```python
from build123d import *

# Parameters (mm, degrees)
SKETCH2_R            = 25
BOSS_EXTRUDE1_DEPTH  = 10
SKETCH3_R            = 20
BOSS_EXTRUDE2_DEPTH  = 8
BOSS_EXTRUDE3_DEPTH  = 20
SKETCH5_R            = 12.5
CUT_EXTRUDE1_DEPTH   = 52.903757089
CUT_SWEEP1_PROFILE_R = 0.625


with BuildPart() as part:
    # Sketch2 → Boss-Extrude1 (new body)
    with BuildSketch(Plane.XY):
        Circle(SKETCH2_R)
    extrude(amount=BOSS_EXTRUDE1_DEPTH)

    # Sketch3 → Boss-Extrude2 (add)
    with BuildSketch(Plane.XY.offset(10)):
        Circle(SKETCH3_R)
    extrude(amount=BOSS_EXTRUDE2_DEPTH)

    # Sketch4 → Boss-Extrude3 (add)
    with BuildSketch(Plane(origin=(0, 0, 0), x_dir=(-1, 0, 0), z_dir=(0, 0, -1))):
        Polygon((-20.437108974, -9.047000469), (-2.383622252, -22.222555786), (18.053486721, -13.175555316), (20.437108974, 9.047000469), (2.383622252, 22.222555786), (-18.053486721, 13.175555316), align=None)
    extrude(amount=BOSS_EXTRUDE3_DEPTH)

    # Sketch5 → Cut-Extrude1 (cut, through all)
    with BuildSketch(Plane(origin=(0, 0, -20), x_dir=(-1, 0, 0), z_dir=(0, 0, -1))):
        Circle(SKETCH5_R)
    extrude(amount=-CUT_EXTRUDE1_DEPTH, mode=Mode.SUBTRACT)

    # Cut-Sweep1: sweep along a path in Sketch6
    with BuildLine(Plane.XY.offset(10)) as cut_sweep1_path:
        CenterArc((0, 0), 23, 0, 360)
    # Cut-Sweep1 profile (on start of the path) → Cut-Sweep1 (sweep, cut)
    with BuildSketch(Plane(origin=(23, 0, 10), x_dir=(0, 0, 1), z_dir=(0, 1, 0))):
        Circle(CUT_SWEEP1_PROFILE_R)
    sweep(path=cut_sweep1_path.line, mode=Mode.SUBTRACT)


solid = part.part
```
For this review, take the finished solid that the model builds, in its own axes (mm). A direction names the side the tool comes from. Coordinates: 2 decimals unless noted, no trailing zeros. Write each loop counter-clockwise with the first axis right and the second up, starting at its lowest first coordinate (ties: lowest second). Pieces come first, ordered by that corner, then holes. Notation, with made-up numbers: (-37.5, -30.5) - (-29.5, -30.5) arc R23 ccw to (-29.5, 3.5) - close; hole circle Ø2 at (65, 58.5). An arc over 180 degrees is marked (long way). Answer in a Markdown table with one row per item. Add a question column.
Q1. We need section B-B, the plane x = 0. State the section outline as (y, z) points (3 decimals), and give its area (3 significant figures).
Q2. We need section C-C, the plane y = 0. State the section outline as (x, z) points (3 decimals), and give its area (3 significant figures).
Q3. Draft analysis for pull direction Y (two halves, no side actions). For faces 1 (the flat face through (7.692, 17.762, -9.86)), 2 (the cylindrical face through (-11.923, 3.755, -1.266)), 3 (the flat face through (-17, -11, 10)), state which applies: +Y half, -Y half, draft (parallel to the pull), parting line (faces both ways), or undercut.
Q4. We need section A-A, the plane z = -9.5. State the section outline as (x, y) points, and give its area (3 significant figures).
Q5. For P1, Ø4, axis at x = 18, z = 5, coming from the +Y side; P2, Ø12, axis at y = -4, z = -15.5, coming from the -X side; P3, Ø10, axis at x = -11, z = -1.5, coming from the +Y side, all flat-tipped, find the tip position at first contact; note any pin that passes through.
Q6. For probe 1 along Y at (x, z) = (0, 7.5); probe 2 along X at (y, z) = (-6.5, -3.5); probe 3 along Y at (x, z) = (0, -11), list the stretches that pass through material, from the lowest coordinate up.
Q7. Tool access review of faces 4 (the flat face through (-11.54, 15.54, -9.86)), 5 (the flat face through (-19.23, -2.22, -9.86)), 6 (the flat face through (13, -15, 0)): name each direction out of +Z, -Z, +X, -X, +Y, -Y from which nothing blocks a thin tool from reaching the whole face with its end or side.
Answer list:
| question | item | result |
|---|---|---|
| 1 | outline | (-25, 0) - (-21.167, 0) - (-21.167, -20) - (-12.5, -20) - (-12.5, 18) - (-20, 18) - (-20, 10) - (-22.375, 10) arc R0.625 cw to (-23.625, 10) - (-25, 10) - close; (12.5, -20) - (21.167, -20) - (21.167, 0) - (25, 0) - (25, 10) - (23.625, 10) arc R0.625 cw to (22.375, 10) - (20, 10) - (20, 18) - (12.5, 18) - close |
| 1 | area | 715 mm2 |
| 2 | outline | (-25, 0) - (-19.467, 0) - (-19.467, -20) - (-12.5, -20) - (-12.5, 18) - (-20, 18) - (-20, 10) - (-22.375, 10) arc R0.625 cw to (-23.625, 10) - (-25, 10) - close; (12.5, -20) - (19.467, -20) - (19.467, 0) - (25, 0) - (25, 10) - (23.625, 10) arc R0.625 cw to (22.375, 10) - (20, 10) - (20, 18) - (12.5, 18) - close |
| 2 | area | 647 mm2 |
| 3 | face 1 | +Y half |
| 3 | face 2 | undercut |
| 3 | face 3 | draft |
| 4 | outline | (-20.44, 9.05) - (-18.05, -13.18) - (2.38, -22.22) - (20.44, -9.05) - (18.05, 13.18) - (-2.38, 22.22) - close; hole circle Ø25 at (0, 0) |
| 4 | area | 807 mm2 |
| 5 | P1 | stops at y = 19.21 |
| 5 | P2 | stops at x = -19.68 |
| 5 | P3 | stops at y = 24.21 |
| 6 | probe 1 | y = -25 to -12.5, 12.5 to 25 |
| 6 | probe 2 | x = -18.77 to -10.68, 10.68 to 20.16 |
| 6 | probe 3 | y = -21.17 to -12.5, 12.5 to 21.17 |
| 7 | face 4 | -Z, -X, +Y |
| 7 | face 5 | -Z, -X, -Y |
| 7 | face 6 | -Z |
